Verification items for the finished model (mm, model axes). A direction names the side the tool comes from. Round coordinates to 2 decimals unless told otherwise and drop trailing zeros. Order: outer loops, then holes, each group sorted by start corner. A loop starts at its lowest first (then second) coordinate and runs counter-clockwise, first axis right, second up. Notation, with made-up numbers: (7.25, 50) -> (49.25, 50) arc R12 ccw to (49.25, 55) -> close; hole circle Ø10 at (76, -20). An arc over 180 degrees is marked (long way). Put each result on its own line as item: value.
from build123d import *

# Parameters (mm, degrees)
PAD_DEPTH           = 6
PAD001_DEPTH        = 10
HOLE_D              = 6
HOLE_DEPTH          = 25
HOLE_CSINK_D        = 12
HOLE_CSINK_ANGLE    = 90
LINEARPATTERN_COUNT = 2
LINEARPATTERN_PITCH = 16


with BuildPart() as part:
    # Sketch → Pad (new body)
    with BuildSketch(Plane.XY):
        with BuildLine():
            Line((-22.5, 0), (22.5, 0))
            Line((22.5, 0), (22.5, 50))
            ThreePointArc((22.5, 50), (19.863961, 56.363961), (13.5, 59))
            Line((13.5, 59), (13.5, 34))
            Line((13.5, 34), (-13.5, 34))
            Line((-13.5, 34), (-13.5, 59))
            ThreePointArc((-13.5, 59), (-19.863961, 56.363961), (-22.5, 50))
            Line((-22.5, 50), (-22.5, 0))
        make_face()
    extrude(amount=PAD_DEPTH)

    # Sketch001 (on Face10 of Pad) → Pad001 (join)
    with BuildSketch(Plane.XY.offset(6)):
        with BuildLine():
            Line((-18, 0), (18, 0))
            Line((18, 0), (18, 34))
            Line((18, 57.794229), (18, 34))
            ThreePointArc((18, 57.794229), (15.829371, 58.693332), (13.5, 59))
            Line((13.5, 34), (13.5, 59))
            Line((-13.5, 34), (13.5, 34))
            Line((-13.5, 59), (-13.5, 34))
            ThreePointArc((-13.5, 59), (-15.829371, 58.693332), (-18, 57.794229))
            Line((-18, 57.794229), (-18, 34))
            Line((-18, 34), (-18, 0))
        make_face()
    extrude(amount=PAD001_DEPTH)

    # Hole
    with Locations(Plane(origin=(0, 0, 0), x_dir=(1, 0, 0), z_dir=(0, 0, -1))):
        with Locations((0, -9)):
            hole = CounterSinkHole(HOLE_D / 2, HOLE_CSINK_D / 2, depth=HOLE_DEPTH, counter_sink_angle=HOLE_CSINK_ANGLE)

    # LinearPattern: Hole ×2
    with Locations(*[(0, i * LINEARPATTERN_PITCH, 0) for i in range(1, LINEARPATTERN_COUNT)]):
        add(hole, mode=Mode.SUBTRACT)


solid = part.part
Item 1: Tool access check on faces 5 (the flat face through (13.5, 46, 8)), 6 (the flat face through (-22.5, 25, 3)), 7 (the flat face through (-18, 29, 11)), 8 (the flat face through (18, 28, 11)). Record the directions out of +Z, -Z, +X, -X, +Y, -Y that give a thin tool (end or side, any length) a straight path to the whole face; none if there is none.
Check sheet entries:
face 5: +Z, -Z, +Y
face 6: +Z, -Z, -X, +Y, -Y
face 7: +Z, -X, +Y, -Y
face 8: +Z, +X, +Y, -Y
Item 2: Gauge pin test, flat ends, axial feed: pin 1 Ø6 at (y, z) = (52, 5) entering from -X; pin 2 Ø5 at (y, z) = (45.5, 10.5) entering from -X; pin 3 Ø3.5 at (x, y) = (-21.5, 18) entering from +Z; pin 4 Ø5 at (x, z) = (3, 9.5) entering from +Y. Record the tip position at first contact, or that the pin passes through.
Check sheet entries:
pin 1: stops at x = -22.5
pin 2: stops at x = -18
pin 3: stops at z = 6
pin 4: stops at y = 34
Item 3: Material ranges on L1, parallel to Y at x = 0, z = 12.25; L2, parallel to X at y = 9, z = 12.25; L3, parallel to Z at x = -20, y = 16.5, recorded low to high. Write a range as [from, to].
Check sheet entries:
L1: y = [0, 6], [12, 22], [28, 34]
L2: x = [-18, -3], [3, 18]
L3: z = [0, 6]
Item 4: Section check B-B on z = 12.5. Record the boundary of the cut face in (x, y), then the cut area to 3 significant figures.
Check sheet entries:
outline: (-18, 0) -> (18, 0) -> (18, 57.79) arc R9 ccw to (13.5, 59) -> (13.5, 34) -> (-13.5, 34) -> (-13.5, 59) arc R9 ccw to (-18, 57.79) -> close; hole circle Ø6 at (0, 9); hole circle Ø6 at (0, 25)
area: 1,390 mm^2
Item 5: Release check for a two-part mould opening along X. For faces 1 (the flat face through (0, 34, 8)), 2 (the flat face through (5, 30, 0)), 3 (the cylindrical face through (-15.8, 58.7, 10.9)), 4 (the cylindrical face through (19.934, 56.294, 2.958)) record: +X half, -X half, draft (parallel to the pull), parting line (faces both ways), or undercut.
Check sheet entries:
face 1: undercut
face 2: draft
face 3: -X half
face 4: +X half
Item 6: Section check A-A on y = 25. Record the boundary of the cut face in (x, z).
Check sheet entries:
outline: (-22.5, 0) -> (-6, 0) -> (-3, 3) -> (-3, 16) -> (-18, 16) -> (-18, 6) -> (-22.5, 6) -> close; (3, 3) -> (6, 0) -> (22.5, 0) -> (22.5, 6) -> (18, 6) -> (18, 16) -> (3, 16) -> close
Item 7: Section check C-C on x = 0. Record the boundary of the cut face in (y, z).
Check sheet entries:
outline: (0, 0) -> (3, 0) -> (6, 3) -> (6, 16) -> (0, 16) -> close; (12, 3) -> (15, 0) -> (19, 0) -> (22, 3) -> (22, 16) -> (12, 16) -> close; (28, 3) -> (31, 0) -> (34, 0) -> (34, 16) -> (28, 16) -> close
Item 8: Section check D-D on z = 5.25. Record the boundary of the cut face in (x, y).
Check sheet entries:
outline: (-22.5, 0) -> (22.5, 0) -> (22.5, 50) arc R9 ccw to (13.5, 59) -> (13.5, 34) -> (-13.5, 34) -> (-13.5, 59) arc R9 ccw to (-22.5, 50) -> close; hole circle Ø6 at (0, 9); hole circle Ø6 at (0, 25)
